Input: part model. Units: mm. Frame: model coordinates. A direction names the side the tool comes from. Coordinates: 2 decimals unless noted, no trailing zeros. Order: outer loops, then holes, each group sorted by start corner. A loop starts at its lowest first (then second) coordinate and runs counter-clockwise, first axis right, second up.
from build123d import *

# Parameters (mm, degrees)
SKETCH1_W           = 26.66
SKETCH1_H           = 79.98
BOSS_EXTRUDE1_DEPTH = 5.08
SKETCH2_W           = 3.81
SKETCH2_H           = 5.08
BOSS_EXTRUDE2_DEPTH = 5.08


with BuildPart() as part:
    # Sketch1 → Boss-Extrude1 (new body)
    with BuildSketch(Plane.XY):
        with Locations((3.269622642, -11.770641509)):
            Rectangle(SKETCH1_W, SKETCH1_H)
    extrude(amount=BOSS_EXTRUDE1_DEPTH)

    # Sketch2 → Boss-Extrude2 (add)
    with BuildSketch(Plane.XY.offset(5.08)):
        with Locations((-1.175377358, -54.300641509)):
            Rectangle(SKETCH2_W, SKETCH2_H)
        with Locations((7.714622642, 30.759358491)):
            Rectangle(SKETCH2_W, SKETCH2_H)
        with Locations((-1.175377358, 30.759358491)):
            Rectangle(SKETCH2_W, SKETCH2_H)
        with Locations((7.714622642, -54.300641509)):
            Rectangle(SKETCH2_W, SKETCH2_H)
    extrude(amount=-BOSS_EXTRUDE2_DEPTH)


solid = part.part
Item 1: Draft query along X for faces 5 (the face through (0.73, 31, 3)), 6 (the face through (8, 33.299, 3)), 7 (the face through (9.62, 31, 3)). Return one class per face: pulls with the +X half, pulls with the -X half, needs draft (parallel to the pull), parting line crosses it, or undercut.
Response values:
face 5: undercut
face 6: needs draft
face 7: pulls with the +X half
Item 2: Cut plane A-A on z = 2.3. Return loops of the section in (x, y), then the cut area to 3 significant figures.
Response values:
outline: (-10.06, -51.76) - (-3.08, -51.76) - (-3.08, -56.84) - (0.73, -56.84) - (0.73, -51.76) - (5.81, -51.76) - (5.81, -56.84) - (9.62, -56.84) - (9.62, -51.76) - (16.6, -51.76) - (16.6, 28.22) - (9.62, 28.22) - (9.62, 33.3) - (5.81, 33.3) - (5.81, 28.22) - (0.73, 28.22) - (0.73, 33.3) - (-3.08, 33.3) - (-3.08, 28.22) - (-10.06, 28.22) - close
area: 2,210 mm2
Item 3: Access query for faces 1 (the face through (5.81, 31, 3)), 2 (the face through (9.62, -54, 3)), 3 (the face through (13, 28.219, 3)), 4 (the face through (-7, 28.219, 3)). Directions: +Z, -Z, +X, -X, +Y, -Y. A direction counts if a zero-diameter tool reaches every point of the face in a straight line with its end or side. Return the directions, or none.
Response values:
face 1: +Z, -Z, +Y
face 2: +Z, -Z, +X, -Y
face 3: +Z, -Z, +X, +Y
face 4: +Z, -Z, -X, +Y
Item 4: Ray query, probe 1 along X at (y, z) = (29.5, 3.9); probe 2 along Y at (x, z) = (-8.25, 4.45). Return the intervals inside material, ascending.
Response values:
probe 1: x = -3.08 to 0.73, 5.81 to 9.62
probe 2: y = -51.76 to 28.22
Item 5: Cut plane B-B on x = 1.75. Return loops of the section in (y, z).
Response values:
outline: (-51.76, 0) - (28.22, 0) - (28.22, 5.08) - (-51.76, 5.08) - close
Item 6: Pin query (flat end, axial travel): pin 1 Ø2.5 at (x, z) = (12.5, 2) entering from -Y; pin 2 Ø2.5 at (x, z) = (-5, 3.5) entering from +Y; pin 3 Ø8 at (x, y) = (-2, 0.5) entering from -Z; pin 4 Ø2.5 at (y, z) = (31, 3.5) entering from -X. Return the tip coordinate at first contact, or that it passes through.
Response values:
pin 1: stops at y = -51.76
pin 2: stops at y = 28.22
pin 3: stops at z = 0
pin 4: stops at x = -3.08
